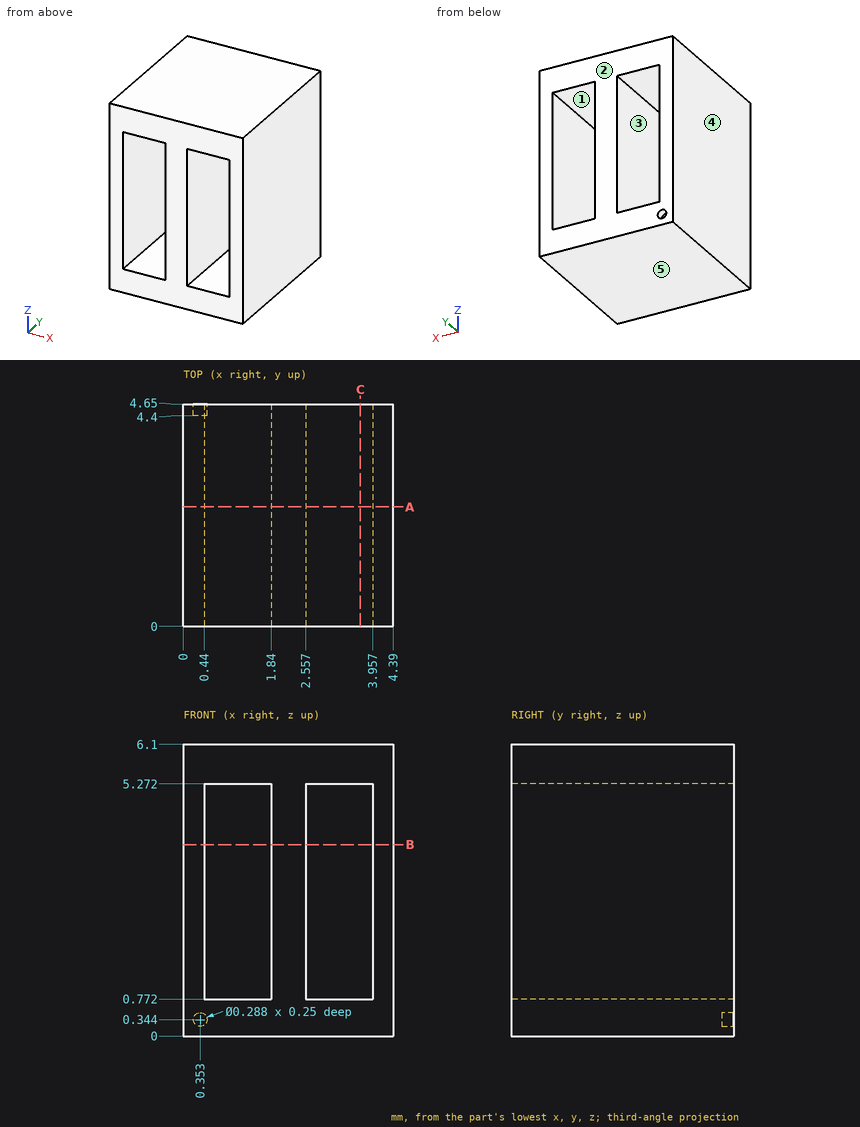
Can you work these out from the drawing? Everything is in mm from the part's minimum corner. A direction names the side the tool comes from. Give positions to 0.01 mm unless a question says otherwise; leave off trailing zeros. Order: outer loops, then holes, each group sorted by start corner. A loop starts at its lowest first (then second) coordinate and runs counter-clockwise, first axis right, second up. Notation, with made-up numbers: M -1.75,26.5 L 25.25,26.5 A11 cw 25.25,33.5 Z; hole C 73.25,67.5 d7. An arc over 180 degrees is marked long. Write item = value, one per line. Start each with the question number.
Q1. Suppose I cut it at C-C (x = 3.7). Write out the boundary of the cut face in (y, z).
Q2. I need wall thicknesses on probe 1 along X at (y, z) = (2.8, 5); probe 2 along Z at (x, y) = (1.6, 2.35). Which ranges of each line are inside material? Lowest first, please. Write a range as [from, to].
Q3. Suppose I cut it at A-A (y = 2.5). Write out the boundary of the cut face in (x, z).
Q4. For the marked faces 1 and 2, which set-ups out of +Z, -Z, +X, -X, +Y, -Y let a thin tool reach every point of the face, with its end or its side?
Q5. Suppose I cut it at B-B (z = 4). Write out the boundary of the cut face in (x, y).
Q6. We'd pull the mould along Z, two halves only. Please class the marked faces 3, 4 and 5: pulls with the +Z half, pulls with the -Z half, needs draft (parallel to the pull), parting line crosses it, or undercut.
Check result:
q1.outline = M 0,0 L 4.65,0 L 4.65,0.77 L 0,0.77 Z; M 0,5.27 L 4.65,5.27 L 4.65,6.1 L 0,6.1 Z
q2.probe_1 = [0, 0.44], [1.84, 2.56], [3.96, 4.39]
q2.probe_2 = [0, 0.77], [5.27, 6.1]
q3.outline = M 0,0 L 4.39,0 L 4.39,6.1 L 0,6.1 Z; hole M 0.44,0.77 L 1.84,0.77 L 1.84,5.27 L 0.44,5.27 Z; hole M 2.56,0.77 L 3.96,0.77 L 3.96,5.27 L 2.56,5.27 Z
q4.face_1 = +Y, -Y
q4.face_2 = +Z, -Z, +X, -X, +Y
q5.outline = M 0,0 L 0.44,0 L 0.44,4.65 L 0,4.65 Z; M 1.84,0 L 2.56,0 L 2.56,4.65 L 1.84,4.65 Z; M 3.96,0 L 4.39,0 L 4.39,4.65 L 3.96,4.65 Z
q6.face_3 = undercut
q6.face_4 = needs draft
q6.face_5 = pulls with the -Z half
